For this review, take the finished solid that the model builds, in its own axes (mm). A direction names the side the tool comes from. Coordinates: 2 decimals unless noted, no trailing zeros. Order: outer loops, then holes, each group sorted by start corner. A loop starts at its lowest first (then second) coordinate and runs counter-clockwise, first axis right, second up. Notation, with made-up numbers: (74, 20.5) -> (91, 20.5) arc R38 ccw to (91, 58.5) -> close; hole circle Ø6 at (-12.75, 32.5). An arc over 180 degrees is marked (long way). Return JSON: item names as keys, results as strings. Group by question number.
Item 1: For line 1 along Z through (x, y) = (0, 0.3); line 2 along X through (y, z) = (0.45, 0); line 3 along X through (y, z) = (1, -12), list the stretches that pass through material, from the lowest coordinate up.
Item 2: Machinability: for faces 4 (the flat face through (12, 1, -3.5)), 5 (the flat face through (0, 1, -15.88)), 6 (the flat face through (-3.5, 1.5, -19.4)), 7 (the flat face through (-3.5, 1, 10)), which of the approach directions +Z, -Z, +X, -X, +Y, -Y give a long, thin tool a straight path to every point of the face, cutting with its end or side? Answer none if there is none.
Item 3: Take a section at B-B (y = 2.45). Count the separate pieces of the cut face and the enclosed holes in it, then the cut area to 3 significant figures.
Item 4: Take a section at A-A (z = -8.5). Write out the cut boundary in (x, y).
Item 5: Insertion check: pin 1 (1.5 mm diameter, centred on x = -6.5, y = 1.5, fed in from +Z); pin 2 (2.5 mm diameter, centred on x = 0, z = -19.88, fed in from -Y); pin 3 (1.6 mm diameter, centred on y = 1, z = 10, fed in from -X); pin 4 (1.5 mm diameter, centred on y = 1.5, z = -8, fed in from -X). Each pin has a flat end and moves straight along its axis. Give the tip position at first contact, or say it passes through.
Item 6: Draft analysis for pull direction Z (two halves, no side actions). For faces 1 (the flat face through (-6.25, 1, -4)), 2 (the flat face through (7, 3, -3)), 3 (the cylindrical face through (7.965, 1.521, -17.579)), state which applies: +Z half, -Z half, draft (parallel to the pull), parting line (faces both ways), or undercut.
```python
from build123d import *

# Parameters (mm, degrees)
SKETCH1_R                                      = 3.5
SKETCH1_W                                      = 16.5
SKETCH1_H                                      = 27
SKETCH1_W_2                                    = 12.5
SKETCH1_H_2                                    = 23
BOSS_EXTRUDE1_DEPTH                            = 3
FILLET1_R                                      = 1
CSK_FOR_M3_FLAT_HEAD_MACHINE_SCREW2_AT_2_COUNT = 2
CSK_FOR_M3_FLAT_HEAD_MACHINE_SCREW2_AT_2_PITCH = 30.1
CSK_FOR_M3_FLAT_HEAD_MACHINE_SCREW2_AT_3_COUNT = 2
CSK_FOR_M3_FLAT_HEAD_MACHINE_SCREW2_AT_3_PITCH = 18.712479793
CSK_FOR_M3_FLAT_HEAD_MACHINE_SCREW2_AT_4_COUNT = 2
CSK_FOR_M3_FLAT_HEAD_MACHINE_SCREW2_AT_4_PITCH = 24.934251543


with BuildPart() as part:
    # Sketch1 → Boss-Extrude1 (new body)
    with BuildSketch(Plane(origin=(0, 0, 0), x_dir=(1, 0, 0), z_dir=(0, 1, 0))):
        with BuildLine():
            ThreePointArc((-11.55, 0), (-12.575126266, 2.474873734), (-15.05, 3.5))
            ThreePointArc((-15.05, 3.5), (-18.55, 0), (-15.05, -3.5))
            ThreePointArc((-15.05, -3.5), (-12.575126266, -2.474873734), (-11.55, 0))
        make_face()
        with BuildLine():
            Line((-8.25, -3.5), (-8.25, 3.5))
            Line((-8.25, 3.5), (-15.05, 3.5))
            ThreePointArc((-15.05, 3.5), (-12.575126266, 2.474873734), (-11.55, 0))
            ThreePointArc((-11.55, 0), (-12.575126266, -2.474873734), (-15.05, -3.5))
            Line((-15.05, -3.5), (-8.25, -3.5))
        make_face()
        with Locations((0, -11.12)):
            Circle(SKETCH1_R)
        with Locations((0, 19.88)):
            Circle(SKETCH1_R)
        with Locations((0, 4.38)):
            Rectangle(SKETCH1_W, SKETCH1_H)
        with Locations((0, 4.38)):
            Rectangle(SKETCH1_W_2, SKETCH1_H_2, mode=Mode.SUBTRACT)
        with BuildLine():
            Line((-2.872281323, -9.12), (-3.5, -9.12))
            Line((-3.5, -9.12), (-3.5, -11.12))
            ThreePointArc((-3.5, -11.12), (-3.339385021, -10.071902827), (-2.872281323, -9.12))
        make_face()
        with BuildLine():
            ThreePointArc((2.872281323, -9.12), (0, -7.62), (-2.872281323, -9.12))
            Line((-2.872281323, -9.12), (2.872281323, -9.12))
        make_face()
        with BuildLine():
            Line((2.872281323, -9.12), (-2.872281323, -9.12))
            ThreePointArc((-2.872281323, -9.12), (-3.339385021, -10.071902827), (-3.5, -11.12))
            ThreePointArc((-3.5, -11.12), (0, -14.62), (3.5, -11.12))
            ThreePointArc((3.5, -11.12), (3.339385021, -10.071902827), (2.872281323, -9.12))
        make_face()
        with BuildLine():
            Line((3.5, -9.12), (2.872281323, -9.12))
            ThreePointArc((2.872281323, -9.12), (3.339385021, -10.071902827), (3.5, -11.12))
            Line((3.5, -11.12), (3.5, -9.12))
        make_face()
        with BuildLine():
            ThreePointArc((3.5, 19.88), (3.339385021, 18.831902827), (2.872281323, 17.88))
            Line((2.872281323, 17.88), (3.5, 17.88))
            Line((3.5, 17.88), (3.5, 19.88))
        make_face()
        with BuildLine():
            Line((2.872281323, 17.88), (-2.872281323, 17.88))
            ThreePointArc((-2.872281323, 17.88), (0, 16.38), (2.872281323, 17.88))
        make_face()
        with BuildLine():
            Line((-3.5, 19.88), (-3.5, 17.88))
            Line((-3.5, 17.88), (-2.872281323, 17.88))
            ThreePointArc((-2.872281323, 17.88), (-3.339385021, 18.831902827), (-3.5, 19.88))
        make_face()
        with BuildLine():
            ThreePointArc((-3.5, 19.88), (-3.339385021, 18.831902827), (-2.872281323, 17.88))
            Line((-2.872281323, 17.88), (2.872281323, 17.88))
            ThreePointArc((2.872281323, 17.88), (3.339385021, 18.831902827), (3.5, 19.88))
            ThreePointArc((3.5, 19.88), (0, 23.38), (-3.5, 19.88))
        make_face()
        with BuildLine():
            Line((15.05, 3.5), (8.25, 3.5))
            Line((8.25, 3.5), (8.25, -3.5))
            Line((8.25, -3.5), (15.05, -3.5))
            ThreePointArc((15.05, -3.5), (11.55, 0), (15.05, 3.5))
        make_face()
        with BuildLine():
            ThreePointArc((18.55, 0), (17.524873734, 2.474873734), (15.05, 3.5))
            ThreePointArc((15.05, 3.5), (11.55, 0), (15.05, -3.5))
            ThreePointArc((15.05, -3.5), (17.524873734, -2.474873734), (18.55, 0))
        make_face()
    extrude(amount=BOSS_EXTRUDE1_DEPTH)

    # Fillet1
    fillet1_edges = [part.edges().sort_by_distance(p)[0] for p in [
        (3.5, 1.5, -17.88),
        (8.25, 1.5, -17.88),
        (8.25, 1.5, -3.5),
        (8.25, 1.5, 3.5),
        (8.25, 1.5, 9.12),
        (-8.25, 1.5, 9.12),
        (-8.25, 1.5, 3.5),
        (-8.25, 1.5, -3.5),
        (-8.25, 1.5, -17.88),
        (-3.5, 1.5, -17.88),
    ]]
    fillet(fillet1_edges, radius=FILLET1_R)

    # Sketch2 → CSK for M3 Flat Head Machine Screw2 (revolve, cut)
    with BuildSketch(Plane(origin=(15.05, 3, 0), x_dir=(0, 0, 1), z_dir=(1, 0, 0))):
        Polygon((0, 0), (0, 3), (1.5, 3), (1.5, 1.65), (3.15, 0), align=None)
    csk_for_m3_flat_head_machine_screw2 = revolve(axis=Axis((15.05, 9.35, 0), (0, -1, 0)), mode=Mode.SUBTRACT)

    # CSK for M3 Flat Head Machine Screw2 at 2: CSK for M3 Flat Head Machine Screw2 ×2
    with Locations(*[(-i * CSK_FOR_M3_FLAT_HEAD_MACHINE_SCREW2_AT_2_PITCH, 0, 0) for i in range(1, CSK_FOR_M3_FLAT_HEAD_MACHINE_SCREW2_AT_2_COUNT)]):
        add(csk_for_m3_flat_head_machine_screw2, mode=Mode.SUBTRACT)

    # CSK for M3 Flat Head Machine Screw2 at 3: CSK for M3 Flat Head Machine Screw2 ×2
    with Locations(*[Vector(-0.804276086, 0, 0.594255819) * (i * CSK_FOR_M3_FLAT_HEAD_MACHINE_SCREW2_AT_3_PITCH) for i in range(1, CSK_FOR_M3_FLAT_HEAD_MACHINE_SCREW2_AT_3_COUNT)]):
        add(csk_for_m3_flat_head_machine_screw2, mode=Mode.SUBTRACT)

    # CSK for M3 Flat Head Machine Screw2 at 4: CSK for M3 Flat Head Machine Screw2 ×2
    with Locations(*[Vector(-0.603587398, 0, -0.797296841) * (i * CSK_FOR_M3_FLAT_HEAD_MACHINE_SCREW2_AT_4_PITCH) for i in range(1, CSK_FOR_M3_FLAT_HEAD_MACHINE_SCREW2_AT_4_COUNT)]):
        add(csk_for_m3_flat_head_machine_screw2, mode=Mode.SUBTRACT)


solid = part.part
```
Findings below:
{
 "1": {"line 1": "z = -23.38 to -21.38, -18.38 to -15.88, 7.12 to 9.62, 12.62 to 14.62", "line 2": "x = -18.55 to -16.55, -13.55 to -6.25, 6.25 to 13.55, 16.55 to 18.55", "line 3": "x = -8.25 to -6.25, 6.25 to 8.25"},
 "2": {"face 4": "-Z, +X, +Y, -Y", "face 5": "+Y, -Y", "face 6": "-Z, -X, +Y, -Y", "face 7": "+Z, -X, +Y, -Y"},
 "3": {"separate pieces": "1", "enclosed holes": "5", "area": "274 mm2"},
 "4": {"outline": "(-8.25, 0) -> (-6.25, 0) -> (-6.25, 3) -> (-8.25, 3) -> close; (6.25, 0) -> (8.25, 0) -> (8.25, 3) -> (6.25, 3) -> close"},
 "5": {"pin 1": "stops at z = 9.12", "pin 2": "passes through", "pin 3": "stops at x = -3.5", "pin 4": "stops at x = -8.25"},
 "6": {"face 1": "undercut", "face 2": "draft", "face 3": "-Z half"}
}
